Geometry: final body of the model. Coordinates: model frame, mm. Face numbers are marked on the shaded views. A direction names the side the tool comes from. Coordinates: 2 decimals unless noted, no trailing zeros. Write each loop counter-clockwise with the first axis right and the second up, starting at its lowest first coordinate (ties: lowest second). Pieces come first, ordered by that corner, then holes.
from build123d import *

# Parameters (mm, degrees)
SKETCH_R        = 2.1
PAD_DEPTH       = 12.5
SKETCH001_W     = 43
SKETCH001_H     = 45.8
POCKET_DEPTH    = 7.5
POCKET001_DEPTH = 4
FILLET_R        = 1.5
SKETCH003_R     = 2.1
PAD001_DEPTH    = 0.4


with BuildPart() as part:
    # Sketch → Pad (new body)
    with BuildSketch(Plane.XY):
        Polygon((-23.15, -26.8), (23.15, -26.8), (25.22, -21.850853), (27, -21.850853), (32.5, -18.675426), (32.5, -12.324574), (27, -9.149147), (27, 9.149147), (32.5, 12.324574), (32.5, 18.675426), (27, 21.850853), (-27, 21.850853), (-32.5, 18.675426), (-32.5, 12.324574), (-27, 9.149147), (-27, -9.149147), (-32.5, -12.324574), (-32.5, -18.675426), (-27, -21.850853), (-25.22, -21.850853), align=None)
        with Locations((-27, 15.5)):
            Circle(SKETCH_R, mode=Mode.SUBTRACT)
        with Locations((-27, -15.5)):
            Circle(SKETCH_R, mode=Mode.SUBTRACT)
        with Locations((27, 15.5)):
            Circle(SKETCH_R, mode=Mode.SUBTRACT)
        with Locations((27, -15.5)):
            Circle(SKETCH_R, mode=Mode.SUBTRACT)
        with BuildLine():
            ThreePointArc((12.5, -2), (0, 10.5), (-12.5, -2))
            Line((-12.5, -2), (-12.5, -6))
            ThreePointArc((-12.5, -6), (0, -18.5), (12.5, -6))
            Line((12.5, -2), (12.5, -6))
        make_face(mode=Mode.SUBTRACT)
        with BuildLine():
            ThreePointArc((-13.85, 13.5), (-15.5, 15.15), (-17.15, 13.5))
            Line((-17.15, 13.5), (-17.15, 9.5))
            ThreePointArc((-17.15, 9.5), (-15.5, 7.85), (-13.85, 9.5))
            Line((-13.85, 13.5), (-13.85, 9.5))
        make_face(mode=Mode.SUBTRACT)
        with BuildLine():
            ThreePointArc((17.15, 13.5), (15.5, 15.15), (13.85, 13.5))
            Line((13.85, 13.5), (13.85, 9.5))
            ThreePointArc((13.85, 9.5), (15.5, 7.85), (17.15, 9.5))
            Line((17.15, 13.5), (17.15, 9.5))
        make_face(mode=Mode.SUBTRACT)
        with BuildLine():
            ThreePointArc((-13.85, -17.5), (-15.5, -15.85), (-17.15, -17.5))
            Line((-17.15, -17.5), (-17.15, -21.5))
            ThreePointArc((-17.15, -21.5), (-15.5, -23.15), (-13.85, -21.5))
            Line((-13.85, -17.5), (-13.85, -21.5))
        make_face(mode=Mode.SUBTRACT)
        with BuildLine():
            ThreePointArc((17.15, -17.5), (15.5, -15.85), (13.85, -17.5))
            Line((13.85, -17.5), (13.85, -21.5))
            ThreePointArc((13.85, -21.5), (15.5, -23.15), (17.15, -21.5))
            Line((17.15, -17.5), (17.15, -21.5))
        make_face(mode=Mode.SUBTRACT)
    extrude(amount=PAD_DEPTH)

    # Sketch001 (on Face46 of Pad) → Pocket (cut)
    with BuildSketch(Plane.XY.offset(12.5)):
        with Locations((0, -3.9)):
            Rectangle(SKETCH001_W, SKETCH001_H)
    extrude(amount=-POCKET_DEPTH, mode=Mode.SUBTRACT)

    # Sketch002 (on Face4 of Pocket) → Pocket001 (cut)
    with BuildSketch(Plane(origin=(0, 0, 0), x_dir=(1, 0, 0), z_dir=(0, 0, -1))):
        Polygon((-23.5, 13.479274), (-23.5, 17.520726), (-27, 19.541452), (-30.5, 17.520726), (-30.5, 13.479274), (-27, 11.458548), align=None)
        Polygon((-23.5, -17.520726), (-23.5, -13.479274), (-27, -11.458548), (-30.5, -13.479274), (-30.5, -17.520726), (-27, -19.541452), align=None)
        Polygon((30.5, -17.520726), (30.5, -13.479274), (27, -11.458548), (23.5, -13.479274), (23.5, -17.520726), (27, -19.541452), align=None)
        Polygon((30.5, 13.479274), (30.5, 17.520726), (27, 19.541452), (23.5, 17.520726), (23.5, 13.479274), (27, 11.458548), align=None)
    extrude(amount=-POCKET001_DEPTH, mode=Mode.SUBTRACT)

    # Fillet
    fillet_edges = [part.edges().sort_by_distance(p)[0] for p in [
        (-21.5, 19, 8.75),
        (21.5, 19, 8.75),
    ]]
    fillet(fillet_edges, radius=FILLET_R)

    # Sketch003 (on Face33 of Fillet) → Pad001 (join)
    with BuildSketch(Plane(origin=(0, 0, 4), x_dir=(1, 0, 0), z_dir=(0, 0, -1))):
        with Locations((-27, 15.5)):
            Circle(SKETCH003_R)
        with Locations((27, 15.5)):
            Circle(SKETCH003_R)
        with Locations((-27, -15.5)):
            Circle(SKETCH003_R)
        with Locations((27, -15.5)):
            Circle(SKETCH003_R)
    extrude(amount=-PAD001_DEPTH)


solid = part.part
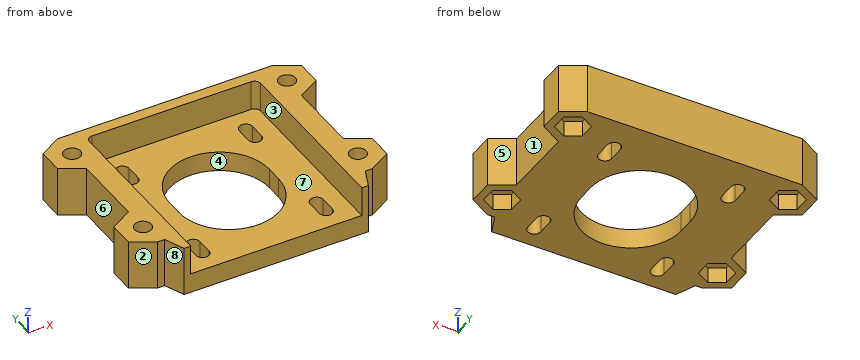
Item 1: Section D-D, the plane x = -15.5. Output: boundary loops of the cut face in (y, z), plus the area to 3 significant figures.
Derived:
outline: (-26.8, 0) - (-23.15, 0) - (-23.15, 5) - (-26.8, 5) - close; (-15.85, 0) - (7.85, 0) - (7.85, 5) - (-15.85, 5) - close; (15.15, 0) - (21.85, 0) - (21.85, 12.5) - (19, 12.5) - (19, 5) - (15.15, 5) - close
area: 192 mm2
Item 2: Material intervals for probe 1 along X at (y, z) = (-15.5, 8.5); probe 2 along X at (y, z) = (3, 9.5); probe 3 along X at (y, z) = (0, 4), sorted ascending.
Derived:
probe 1: x = -32.5 to -29.1, -24.9 to -21.5, 21.5 to 24.9, 29.1 to 32.5
probe 2: x = -27 to -21.5, 21.5 to 27
probe 3: x = -27 to -12.34, 12.34 to 27
Item 3: Section A-A, the plane y = -3.5. Output: boundary loops of the cut face in (x, z), plus the area to 4 significant figures.
Derived:
outline: (-27, 0) - (-12.5, 0) - (-12.5, 5) - (-21.5, 5) - (-21.5, 12.5) - (-27, 12.5) - close; (12.5, 0) - (27, 0) - (27, 12.5) - (21.5, 12.5) - (21.5, 5) - (12.5, 5) - close
area: 227.5 mm2
Item 4: Section C-C, the plane z = 11.25. State how many separate pieces and enclosed holes the cut face has, plus the area to 3 significant figures.
Derived:
separate pieces: 1
enclosed holes: 4
area: 785 mm2
Item 5: Pin query (flat end, axial travel): pin 1 (2.5 mm diameter, centred on x = -27, y = -15.5, fed in from +Z); pin 2 (7.5 mm diameter, centred on x = -26, y = -17.5, fed in from -Z); pin 3 (4 mm diameter, centred on x = 4, z = 10.5, fed in from -Y); pin 4 (4 mm diameter, centred on x = 27, y = -15.5, fed in from -Z). Return the tip coordinate at first contact, or that it passes through.
Derived:
pin 1: stops at z = 4.4
pin 2: stops at z = 0
pin 3: stops at y = 19
pin 4: stops at z = 4
Item 6: Pull-direction query (X, two-part tool) for the marked faces 1, 2 and 3; classes: released by +X, released by -X, zero draft, split by the parting line, or undercut.
Derived:
face 1: released by +X
face 2: released by -X
face 3: undercut
Item 7: Set-up query: the marked faces 4, 5, 6, 7 and 8. Return all of +Z, -Z, +X, -X, +Y, -Y with unobstructed straight access to the full face (end or side cutting, diameter ignored); none if empty.
Derived:
face 4: +Z, -Z
face 5: +Z, -Z, +X
face 6: +Z, -Z, -X
face 7: +Z, -Y
face 8: +Z, -Z, -X, -Y
Item 8: Section B-B, the plane x = 0. Output: boundary loops of the cut face in (y, z), plus the area to 3 significant figures.
Derived:
outline: (-26.8, 0) - (-18.5, 0) - (-18.5, 5) - (-26.8, 5) - close; (10.5, 0) - (21.85, 0) - (21.85, 12.5) - (19, 12.5) - (19, 5) - (10.5, 5) - close
area: 120 mm2
